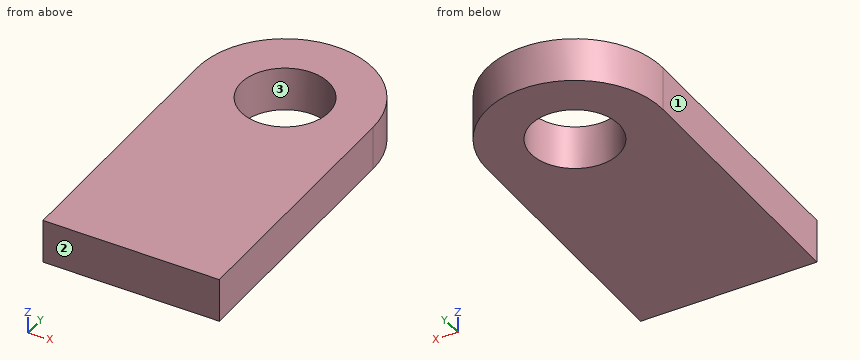
```python
from build123d import *

# Parameters (mm, degrees)
F0_R     = 127
F1_DEPTH = 127


with BuildPart() as f1:
    # F0 (on Top) → F1 (new body)
    with BuildSketch(Plane.XY):
        with BuildLine():
            Line((-254, 0), (-254, -762))
            Line((-254, -762), (254, -762))
            Line((254, -762), (254, 0))
            ThreePointArc((254, 0), (0, 254), (-254, 0))
        make_face()
        Circle(F0_R, mode=Mode.SUBTRACT)
    extrude(amount=F1_DEPTH)


solid = f1.part
```
Work out the finished part from the listing and answer in its coordinate system (mm). Face numbers are marked on the shaded views. Coordinates: 2 decimals unless noted, no trailing zeros. Loops run counter-clockwise (first coordinate to the right, second up) from the corner with the lowest first, then second, coordinate; pieces in that order, holes last. Notation, with made-up numbers: (29, 6.25) -> (85, 6.25) arc R32 cw to (85, 36.25) -> close; hole circle Ø10 at (-15.5, -38.5). An arc over 180 degrees is marked (long way). Answer as CSV lines item,"result".
Q1. Each of these flat-tipped pins is pushed along its axis until it touches: pin 1 (4 mm diameter, centred on x = -175.5, y = -185.5, fed in from -Z); pin 2 (6 mm diameter, centred on x = -111.5, z = 59.5, fed in from +Y); pin 3 (8 mm diameter, centred on x = -144, z = 23.5, fed in from +Y); pin 4 (8 mm diameter, centred on x = -48, z = 87, fed in from +Y). Where does it stop, or does it pass through?
Findings:
pin 1,"stops at z = 0"
pin 2,"stops at y = 229.66"
pin 3,"stops at y = 211.93"
pin 4,"stops at y = 250.16"
Q2. For a pull along X with two mould halves and no side action, classify the marked faces 1, 2 and 3 as +X half, -X half, draft (parallel to the pull), parting line (faces both ways), or undercut.
Findings:
face 1,"-X half"
face 2,"draft"
face 3,"undercut"
Q3. Find the intervals of material crossed by probe 1 along X at (y, z) = (-1.5, 57); probe 2 along Y at (x, z) = (0, 101); probe 3 along Y at (x, z) = (49.5, 18.5), in increasing order.
Findings:
probe 1,"x = -254 to -126.99, 126.99 to 254"
probe 2,"y = -762 to -127, 127 to 254"
probe 3,"y = -762 to -116.96, 116.96 to 249.13"
Q4. The part is cut by section D-D on x = 212. Write down the section's boundary in (y, z).
Findings:
outline,"(-762, 0) -> (139.9, 0) -> (139.9, 127) -> (-762, 127) -> close"
Q5. The part is cut by section C-C on y = -117.5. Write down the section's boundary in (x, z), and give its area (3 significant figures).
Findings:
outline,"(-254, 0) -> (-48.19, 0) -> (-48.19, 127) -> (-254, 127) -> close; (48.19, 0) -> (254, 0) -> (254, 127) -> (48.19, 127) -> close"
area,"52,300 mm²"
Q6. The part is cut by section A-A on x = 0. Write down the section's boundary in (y, z).
Findings:
outline,"(-762, 0) -> (-127, 0) -> (-127, 127) -> (-762, 127) -> close; (127, 0) -> (254, 0) -> (254, 127) -> (127, 127) -> close"
Q7. The part is cut by section B-B on z = 101.5. Write down the section's boundary in (x, y), and give its area (3 significant figures).
Findings:
outline,"(-254, -762) -> (254, -762) -> (254, 0) arc R254 ccw to (-254, 0) -> close; hole circle Ø254 at (0, 0)"
area,"438,000 mm²"
